```python
from build123d import *

# Parameters (mm, degrees)
SKETCH1_R                       = 21.15
BOSS_EXTRUDE1_DEPTH             = 5
SKETCH2_R                       = 21.15
SKETCH2_R_2                     = 19.15
BOSS_EXTRUDE2_DEPTH             = 10
SKETCH3_R                       = 8
SKETCH3_W                       = 53.18
SKETCH3_H                       = 53.18
SKETCH3_W_2                     = 43.18
SKETCH3_H_2                     = 43.18
SKETCH3_R_2                     = 21.15
BOSS_EXTRUDE4_DEPTH             = 5
SKETCH4_W                       = 106.36
SKETCH4_H                       = 53.18
SKETCH4_W_2                     = 43.18
SKETCH4_H_2                     = 43.18
SKETCH4_R                       = 0.5
SKETCH4_R_2                     = 4.25
BOSS_EXTRUDE5_DEPTH             = 55
BOSS_EXTRUDE5_DIRECTION_2_REACH = 97.637
SKETCH5_R                       = 1.566567696
SKETCH5_R_2                     = 1.356312868
SKETCH5_R_3                     = 1.387107712
SKETCH5_R_4                     = 1.945059914
BOSS_EXTRUDE6_DEPTH             = 50
SKETCH6_W                       = 106.36
SKETCH6_H                       = 53.18
SKETCH6_R                       = 3
SKETCH6_R_2                     = 2
BOSS_EXTRUDE7_DEPTH             = 5
SKETCH7_W                       = 22
SKETCH7_H                       = 23
CUT_EXTRUDE1_DEPTH              = 5
BOSS_EXTRUDE8_DEPTH             = 60
BOSS_EXTRUDE9_DEPTH             = 5


with BuildPart() as part:
    # Sketch1 → Boss-Extrude1 (new body)
    with BuildSketch(Plane(origin=(0, 0, 0), x_dir=(1, 0, 0), z_dir=(0, 1, 0))):
        with Locations(Location((0, 0, 0), (0, 0, 270))):
            Circle(SKETCH1_R)
    extrude(amount=BOSS_EXTRUDE1_DEPTH)

    # Sketch2 → Boss-Extrude2 (add)
    with BuildSketch(Plane(origin=(0, 0, 0), x_dir=(1, 0, 0), z_dir=(0, 1, 0))):
        with Locations(Location((0, 0, 0), (0, 0, 270))):
            Circle(SKETCH2_R)
        with Locations(Location((0, 0, 0), (0, 0, 270))):
            Circle(SKETCH2_R_2, mode=Mode.SUBTRACT)
    extrude(amount=BOSS_EXTRUDE2_DEPTH)

    # Sketch3 → Boss-Extrude4 (add)
    with BuildSketch(Plane(origin=(0, 0, 0), x_dir=(1, 0, 0), z_dir=(0, 1, 0))):
        with Locations((31.59, -20)):
            Circle(SKETCH3_R)
        with Locations((-31.59, -20)):
            Circle(SKETCH3_R)
        with Locations((26.59, 52.74)):
            Rectangle(SKETCH3_W, SKETCH3_H)
        with Locations((26.59, 52.74)):
            Rectangle(SKETCH3_W_2, SKETCH3_H_2, mode=Mode.SUBTRACT)
        with Locations((-26.59, 52.74)):
            Rectangle(SKETCH3_W, SKETCH3_H)
        with Locations((-26.59, 52.74)):
            Rectangle(SKETCH3_W_2, SKETCH3_H_2, mode=Mode.SUBTRACT)
        with BuildLine():
            Line((53.18, 26.15), (0, 26.15))
            Line((0, 26.15), (-53.18, 26.15))
            Line((-53.18, 26.15), (-31.59, 13.685007688))
            Line((-31.59, 13.685007688), (-31.59, 0.832649627))
            Line((-31.59, 0.832649627), (-36.793594364, -13.923602573))
            ThreePointArc((-36.793594364, -13.923602573), (-28.245508627, -12.732649901), (-23.59, -20))
            ThreePointArc((-23.59, -20), (-24.322649901, -23.344491373), (-26.386405636, -26.076397427))
            Line((-26.386405636, -26.076397427), (0, -21.15))
            Line((0, -21.15), (26.386405636, -26.076397427))
            ThreePointArc((26.386405636, -26.076397427), (25.513602573, -14.796405636), (36.793594364, -13.923602573))
            Line((36.793594364, -13.923602573), (31.59, 0.832649627))
            Line((31.59, 0.832649627), (31.59, 13.685007688))
            Line((31.59, 13.685007688), (53.18, 26.15))
        make_face()
        with BuildLine():
            ThreePointArc((21.15, 0), (14.955308422, -14.955308422), (0, -21.15))
            ThreePointArc((0, -21.15), (-14.955308422, 14.955308422), (21.15, 0))
        make_face(mode=Mode.SUBTRACT)
        with Locations(Location((0, 0, 0), (0, 0, 270))):
            Circle(SKETCH3_R_2)
    extrude(amount=BOSS_EXTRUDE4_DEPTH)

    # Sketch4 → Boss-Extrude5 (add)
    with BuildSketch(Plane(origin=(0, 5, 0), x_dir=(1, 0, 0), z_dir=(0, 1, 0))):
        with Locations((0, 52.74)):
            Rectangle(SKETCH4_W, SKETCH4_H)
        with Locations((-26.59, 52.74)):
            Rectangle(SKETCH4_W_2, SKETCH4_H_2, mode=Mode.SUBTRACT)
        with Locations((26.59, 52.74)):
            Rectangle(SKETCH4_W_2, SKETCH4_H_2, mode=Mode.SUBTRACT)
        with BuildLine():
            ThreePointArc((-31.59, -12), (-39.59, -20), (-31.59, -28))
            Line((-31.59, -28), (-25.59, -31))
            Line((-25.59, -31), (-22.59, -31))
            Line((-22.59, -31), (-22.59, -9))
            Line((-22.59, -9), (-25.59, -9))
            Line((-25.59, -9), (-31.59, -12))
        make_face()
        with Locations(Location((-25.59, -27.5, 0), (0, 0, 270))):
            Circle(SKETCH4_R, mode=Mode.SUBTRACT)
        with Locations(Location((-31.59, -20, 0), (0, 0, 270))):
            Circle(SKETCH4_R_2, mode=Mode.SUBTRACT)
        with Locations(Location((-25.59, -12.5, 0), (0, 0, 270))):
            Circle(SKETCH4_R, mode=Mode.SUBTRACT)
        with BuildLine():
            Line((31.59, -12), (25.59, -9))
            Line((25.59, -9), (22.59, -9))
            Line((22.59, -9), (22.59, -31))
            Line((22.59, -31), (25.59, -31))
            Line((25.59, -31), (31.59, -28))
            ThreePointArc((31.59, -28), (39.59, -20), (31.59, -12))
        make_face()
        with Locations(Location((25.59, -27.5, 0), (0, 0, 270))):
            Circle(SKETCH4_R, mode=Mode.SUBTRACT)
        with Locations(Location((25.59, -12.5, 0), (0, 0, 270))):
            Circle(SKETCH4_R, mode=Mode.SUBTRACT)
        with Locations(Location((31.59, -20, 0), (0, 0, 270))):
            Circle(SKETCH4_R_2, mode=Mode.SUBTRACT)
    extrude(amount=BOSS_EXTRUDE5_DEPTH)

    # Boss-Extrude5 direction 2: up to this face of the body (flat: up to its plane)
    boss_extrude5_direction_2_end = Plane(part.part.faces().sort_by_distance((0, 0, -18.773899986))[0])
    # Sketch4 → Boss-Extrude5 direction 2 (add, up to the picked face)
    with BuildSketch(Plane(origin=(0, 5, 0), x_dir=(1, 0, 0), z_dir=(0, 1, 0)), mode=Mode.PRIVATE) as boss_extrude5_direction_2_sk1:
        with Locations((0, 52.74)):
            Rectangle(SKETCH4_W, SKETCH4_H)
        with Locations((-26.59, 52.74)):
            Rectangle(SKETCH4_W_2, SKETCH4_H_2, mode=Mode.SUBTRACT)
        with Locations((26.59, 52.74)):
            Rectangle(SKETCH4_W_2, SKETCH4_H_2, mode=Mode.SUBTRACT)
    boss_extrude5_direction_2_tool1 = split(extrude(boss_extrude5_direction_2_sk1.sketch, amount=-BOSS_EXTRUDE5_DIRECTION_2_REACH, mode=Mode.PRIVATE), bisect_by=boss_extrude5_direction_2_end, keep=Keep.BOTH, mode=Mode.PRIVATE)
    # Sketch4 → Boss-Extrude5 direction 2 (add, up to the picked face)
    with BuildSketch(Plane(origin=(0, 5, 0), x_dir=(1, 0, 0), z_dir=(0, 1, 0)), mode=Mode.PRIVATE) as boss_extrude5_direction_2_sk2:
        with BuildLine():
            ThreePointArc((-31.59, -12), (-39.59, -20), (-31.59, -28))
            Line((-31.59, -28), (-25.59, -31))
            Line((-25.59, -31), (-22.59, -31))
            Line((-22.59, -31), (-22.59, -9))
            Line((-22.59, -9), (-25.59, -9))
            Line((-25.59, -9), (-31.59, -12))
        make_face()
        with Locations(Location((-25.59, -27.5, 0), (0, 0, 270))):
            Circle(SKETCH4_R, mode=Mode.SUBTRACT)
        with Locations(Location((-31.59, -20, 0), (0, 0, 270))):
            Circle(SKETCH4_R_2, mode=Mode.SUBTRACT)
        with Locations(Location((-25.59, -12.5, 0), (0, 0, 270))):
            Circle(SKETCH4_R, mode=Mode.SUBTRACT)
    boss_extrude5_direction_2_tool2 = split(extrude(boss_extrude5_direction_2_sk2.sketch, amount=-BOSS_EXTRUDE5_DIRECTION_2_REACH, mode=Mode.PRIVATE), bisect_by=boss_extrude5_direction_2_end, keep=Keep.BOTH, mode=Mode.PRIVATE)
    # Sketch4 → Boss-Extrude5 direction 2 (add, up to the picked face)
    with BuildSketch(Plane(origin=(0, 5, 0), x_dir=(1, 0, 0), z_dir=(0, 1, 0)), mode=Mode.PRIVATE) as boss_extrude5_direction_2_sk3:
        with BuildLine():
            Line((31.59, -12), (25.59, -9))
            Line((25.59, -9), (22.59, -9))
            Line((22.59, -9), (22.59, -31))
            Line((22.59, -31), (25.59, -31))
            Line((25.59, -31), (31.59, -28))
            ThreePointArc((31.59, -28), (39.59, -20), (31.59, -12))
        make_face()
        with Locations(Location((25.59, -27.5, 0), (0, 0, 270))):
            Circle(SKETCH4_R, mode=Mode.SUBTRACT)
        with Locations(Location((25.59, -12.5, 0), (0, 0, 270))):
            Circle(SKETCH4_R, mode=Mode.SUBTRACT)
        with Locations(Location((31.59, -20, 0), (0, 0, 270))):
            Circle(SKETCH4_R_2, mode=Mode.SUBTRACT)
    boss_extrude5_direction_2_tool3 = split(extrude(boss_extrude5_direction_2_sk3.sketch, amount=-BOSS_EXTRUDE5_DIRECTION_2_REACH, mode=Mode.PRIVATE), bisect_by=boss_extrude5_direction_2_end, keep=Keep.BOTH, mode=Mode.PRIVATE)
    add(boss_extrude5_direction_2_tool1.solids().sort_by(Axis((0, 5, -52.74), (0, -1, 0)))[0])
    add(boss_extrude5_direction_2_tool2.solids().sort_by(Axis((-39.311971, 5, 20), (0, -1, 0)))[0])
    add(boss_extrude5_direction_2_tool3.solids().sort_by(Axis((28.465662, 5, 10.748676), (0, -1, 0)))[0])

    # Sketch5 → Boss-Extrude6 (add)
    with BuildSketch(Plane(origin=(0, 5, 0), x_dir=(1, 0, 0), z_dir=(0, 1, 0))):
        with Locations((-25.59, -27.5)):
            Circle(SKETCH5_R)
        with Locations((-25.59, -12.5)):
            Circle(SKETCH5_R_2)
        with Locations((25.59, -12.5)):
            Circle(SKETCH5_R_3)
        with Locations((25.59, -23.409830044)):
            Circle(SKETCH5_R_4)
    extrude(amount=BOSS_EXTRUDE6_DEPTH)

    # Sketch6 → Boss-Extrude7 (add)
    with BuildSketch(Plane(origin=(0, 60, 0), x_dir=(1, 0, 0), z_dir=(0, 1, 0))):
        with Locations((0, 52.74)):
            Rectangle(SKETCH6_W, SKETCH6_H)
        with Locations(Location((-26.59, 52.74, 0), (0, 0, 270))):
            Circle(SKETCH6_R, mode=Mode.SUBTRACT)
        with Locations(Location((26.59, 52.74, 0), (0, 0, 270))):
            Circle(SKETCH6_R, mode=Mode.SUBTRACT)
        with Locations(Location((-42.09, 68.24, 0), (0, 0, 270))):
            Circle(SKETCH6_R_2, mode=Mode.SUBTRACT)
        with Locations(Location((-11.09, 68.24, 0), (0, 0, 270))):
            Circle(SKETCH6_R_2, mode=Mode.SUBTRACT)
        with Locations(Location((-11.09, 37.24, 0), (0, 0, 270))):
            Circle(SKETCH6_R_2, mode=Mode.SUBTRACT)
        with Locations(Location((-42.09, 37.24, 0), (0, 0, 270))):
            Circle(SKETCH6_R_2, mode=Mode.SUBTRACT)
        with Locations(Location((11.09, 68.24, 0), (0, 0, 90))):
            Circle(SKETCH6_R_2, mode=Mode.SUBTRACT)
        with Locations(Location((11.09, 37.24, 0), (0, 0, 90))):
            Circle(SKETCH6_R_2, mode=Mode.SUBTRACT)
        with Locations(Location((42.09, 37.24, 0), (0, 0, 90))):
            Circle(SKETCH6_R_2, mode=Mode.SUBTRACT)
        with Locations(Location((42.09, 68.24, 0), (0, 0, 90))):
            Circle(SKETCH6_R_2, mode=Mode.SUBTRACT)
    extrude(amount=BOSS_EXTRUDE7_DEPTH)

    # Sketch7 → Cut-Extrude1 (cut)
    with BuildSketch(Plane(origin=(0, 0, -79.33), x_dir=(-1, 0, 0), z_dir=(0, 0, -1))):
        with Locations((-28.18, 11.5)):
            Rectangle(SKETCH7_W, SKETCH7_H)
        with Locations((28.18, 11.5)):
            Rectangle(SKETCH7_W, SKETCH7_H)
    extrude(amount=-CUT_EXTRUDE1_DEPTH, mode=Mode.SUBTRACT)

    # Sketch8 → Boss-Extrude8 (add)
    with BuildSketch(Plane(origin=(0, 60, 0), x_dir=(1, 0, 0), z_dir=(0, 1, 0))):
        Polygon((-31.542803854, -13.152023689), (-31.542803854, 26.15), (-22.59, 26.15), (-22.59, -9.877338884), (-22.59, -11.171477367), align=None)
        Polygon((31.542803854, 26.15), (22.59, 26.15), (22.59, -9.877338884), (22.59, -11.171477367), (31.542803854, -13.152023689), align=None)
    extrude(amount=-BOSS_EXTRUDE8_DEPTH)

    # Sketch9 → Boss-Extrude9 (add)
    with BuildSketch(Plane(origin=(0, 5, 0), x_dir=(1, 0, 0), z_dir=(0, 1, 0))):
        with BuildLine():
            Line((-22.59, -25.36760051), (-22.59, -31))
            Line((-22.59, -31), (-2.93570785, -24.964116951))
            ThreePointArc((-2.93570785, -24.964116951), (0, -24.523490331), (2.93570785, -24.964116951))
            Line((2.93570785, -24.964116951), (22.59, -31))
            Line((22.59, -31), (22.59, -25.36760051))
            Line((22.59, -25.36760051), (0, -21.15))
            Line((0, -21.15), (-22.59, -25.36760051))
        make_face()
    extrude(amount=-BOSS_EXTRUDE9_DEPTH)


solid = part.part
```
CAD build for the part. Positions are in the model's coordinates, mm. A direction names the side the tool comes from. Coordinates: 2 decimals unless noted, no trailing zeros. Order: outer loops, then holes, each group sorted by start corner. A loop starts at its lowest first (then second) coordinate and runs counter-clockwise, first axis right, second up. Notation, with made-up numbers: (-20.5, 4) - (-8.5, 4) arc R23 cw to (-8.5, 19) - close; hole circle Ø1 at (-9.75, -39.75). An arc over 180 degrees is marked (long way). Use a Markdown table: item, result. Add a question column.
(1) Saw through at D-D (z = -52.74). Give the cut face in (x, y), then the cut area to 3 significant figures.
(2) Which spindle directions (+Z, -Z, +X, -X, +Y, -Y) get a long thin tool onto all of the face, cutting with end or side? Do faces 1 (the face through (-39.588, 29.58, 19.824)), 2 (the face through (-5, 30, -52)), 3 (the face through (5.752, 7.465, 18.266)), 4 (the face through (-27, 60, 2)). Say none if no direction does.
(3) Saw through at A-A (z = -68.24). Give the cut face in (x, y), then the cut area to 3 significant figures.
(4) Saw through at C-C (x = -34). Give the cut face in (y, z), then the cut area to 3 significant figures.
(5) Pull direction X, two halves, no side cores. Call faces 5 (the face through (-34, 2, 6)), 6 (the face through (40.7, 62.5, -66.8)), 7 (the face through (24, 30, 31)): +X half, -X half, draft (parallel to the pull), parting line (faces both ways), or undercut.
(6) Drill centre lines: line 1 along X through (y, z) = (63.9, -37.24); line 2 along X through (y, z) = (62.15, -52.74); line 3 along X through (y, z) = (3.5, -73). Where is each one in solid material? Low to high. Write a range as [from, to].
(7) Flat gauge pins, fed straight in: pin 1 (18 mm diameter, centred on x = 9.5, y = 20.5, fed in from +Z); pin 2 (6 mm diameter, centred on x = -12.5, z = -58, fed in from -Y); pin 3 (13 mm diameter, centred on x = -31, y = 15.5, fed in from -Z); pin 4 (3 mm diameter, centred on x = 11.09, z = -68.24, fed in from -Y). Where does each tip first touch, or does it go through?
(8) Saw through at B-B (y = 53). Count the separate pieces of the cut face and the enclosed holes in it, then the cut area to 3 significant figures.
Solved:
| question | item | result |
|---|---|---|
| 1 | outline | (-53.18, 0) - (-48.18, 0) - (-48.18, 60) - (-29.59, 60) - (-29.59, 65) - (-53.18, 65) - close; (-23.59, 60) - (-5, 60) - (-5, 0) - (5, 0) - (5, 60) - (23.59, 60) - (23.59, 65) - (-23.59, 65) - close; (29.59, 60) - (48.18, 60) - (48.18, 0) - (53.18, 0) - (53.18, 65) - (29.59, 65) - close |
| 1 | area | 1,670 mm² |
| 2 | face 1 | -X, +Y |
| 2 | face 2 | -Y |
| 2 | face 3 | +Y |
| 2 | face 4 | +Z, +X, -X, +Y |
| 3 | outline | (-53.18, 0) - (-48.18, 0) - (-48.18, 60) - (-44.09, 60) - (-44.09, 65) - (-53.18, 65) - close; (-40.09, 60) - (-13.09, 60) - (-13.09, 65) - (-40.09, 65) - close; (-9.09, 60) - (-5, 60) - (-5, 0) - (5, 0) - (5, 60) - (9.09, 60) - (9.09, 65) - (-9.09, 65) - close; (13.09, 60) - (40.09, 60) - (40.09, 65) - (13.09, 65) - close; (44.09, 60) - (48.18, 60) - (48.18, 0) - (53.18, 0) - (53.18, 65) - (44.09, 65) - close |
| 3 | area | 1,650 mm² |
| 4 | outline | (0, -31.15) - (60, -31.15) - (60, -74.33) - (23, -74.33) - (23, -79.33) - (65, -79.33) - (65, -26.15) - (5, -26.15) - (5, -15.08) - (0, -15.08) - close; (0, 6) - (5, 6) - (5, 12.37) - (60, 12.37) - (60, 16.5) - (5, 16.5) - (5, 23.5) - (60, 23.5) - (60, 27.63) - (0, 27.63) - close |
| 4 | area | 1,370 mm² |
| 5 | face 5 | -X half |
| 5 | face 6 | undercut |
| 5 | face 7 | draft |
| 6 | line 1 | x = [-53.18, -44.09], [-40.09, -13.09], [-9.09, 9.09], [13.09, 40.09], [44.09, 53.18] |
| 6 | line 2 | x = [-53.18, -29.59], [-23.59, 23.59], [29.59, 53.18] |
| 6 | line 3 | x = [-53.18, -48.18], [-5, 5], [48.18, 53.18] |
| 7 | pin 1 | stops at z = -26.15 |
| 7 | pin 2 | stops at y = 60 |
| 7 | pin 3 | stops at z = -31.15 |
| 7 | pin 4 | passes through |
| 8 | separate pieces | 1 |
| 8 | enclosed holes | 5 |
| 8 | area | 3,020 mm² |
